from build123d import *

# Parameters (mm, degrees)
SKETCH_2_R          = 1.67
CUT_EXTRUDE_1_DEPTH = 10.939185077


with BuildPart() as part:
    # 草图1 → 旋转1 (revolve)
    with BuildSketch(Plane.XY, mode=Mode.PRIVATE) as revolve_1_sk:
        Polygon((0, 0), (3.12, 0), (3.12, 5.36), (3.93, 5.36), (3.93, 6.14), (3.12, 6.14), (3.12, 8.24), (0, 8.24), align=None)
    revolve(revolve_1_sk.sketch.rotate(Axis((0, 0, 0), (0, 1, 0)), 90), axis=Axis((0, 0, 0), (0, 1, 0)))

    # 草图2 → 切除-拉伸1 (cut, through all)
    with BuildSketch(Plane.XZ):
        with Locations(Location((0, 0, 0), (0, 0, 270))):
            Circle(SKETCH_2_R)
    extrude(amount=-CUT_EXTRUDE_1_DEPTH, mode=Mode.SUBTRACT)

    # 草图4 → 切除-旋转1 (revolve, cut)
    with BuildSketch(Plane.XY, mode=Mode.PRIVATE) as cut_revolve_1_sk:
        Polygon((2.62, 0), (1.67, 0.95), (0, 0.95), (0, 0), align=None)
        Polygon((2.62, 8.24), (1.67, 7.29), (0, 7.29), (0, 8.24), align=None)
    revolve(cut_revolve_1_sk.sketch.rotate(Axis((0, 0, 0), (0, -1, 0)), 90), axis=Axis((0, 0, 0), (0, -1, 0)), mode=Mode.SUBTRACT)


solid = part.part
Verification items for the finished model (mm, model axes). A direction names the side the tool comes from. Give positions to 0.01 mm unless a question says otherwise; leave off trailing zeros. Loops run counter-clockwise (first coordinate to the right, second up) from the corner with the lowest first, then second, coordinate; pieces in that order, holes last.
1. Cross-section at D-D on x = 2.75. Record the cut outline in (y, z).
Derived:
outline: (0, -1.47) - (5.36, -1.47) - (5.36, -2.81) - (6.14, -2.81) - (6.14, -1.47) - (8.24, -1.47) - (8.24, 1.47) - (6.14, 1.47) - (6.14, 2.81) - (5.36, 2.81) - (5.36, 1.47) - (0, 1.47) - close
2. Tool access check on faces 1 (the flat face through (-2, 8.24, 2)), 2 (the cylindrical face through (-0.937, 7.205, -2.976)), 3 (the cylindrical face through (-0.937, 2.718, -2.976)). Record the directions out of +Z, -Z, +X, -X, +Y, -Y that give a thin tool (end or side, any length) a straight path to the whole face; none if there is none.
Derived:
face 1: +Z, -Z, +X, -X, +Y
face 2: +Y
face 3: -Y
3. Release check for a two-part mould opening along Z. For faces 4 (the cylindrical face through (3.837, 5.755, 0.852)), 5 (the flat face through (-2, 0, -2)), 6 (the cylindrical face through (0.502, 4.076, -1.593)) record: +Z half, -Z half, draft (parallel to the pull), parting line (faces both ways), or undercut.
Derived:
face 4: parting line
face 5: draft
face 6: undercut
4. Cross-section at A-A on x = 0. Record the cut outline in (y, z), and give its area (3 significant figures).
Derived:
outline: (0, -3.12) - (5.36, -3.12) - (5.36, -3.93) - (6.14, -3.93) - (6.14, -3.12) - (8.24, -3.12) - (8.24, -2.62) - (7.29, -1.67) - (0.95, -1.67) - (0, -2.62) - close; (0, 2.62) - (0.95, 1.67) - (7.29, 1.67) - (8.24, 2.62) - (8.24, 3.12) - (6.14, 3.12) - (6.14, 3.93) - (5.36, 3.93) - (5.36, 3.12) - (0, 3.12) - close
area: 23.4 mm2
5. Go/stop test with flat-tipped pins: P1, Ø4, axis at x = 0, z = 0, coming from the -Y side; P2, Ø2, axis at x = -1, y = 2, coming from the -Z side; P3, Ø4, axis at x = 0, z = -0.5, coming from the -Y side. Record where each tip stops, or that it passes through.
Derived:
P1: stops at y = 0.62
P2: stops at z = -3.12
P3: stops at y = 0.12
6. Cross-section at B-B on z = 0. Record the cut outline in (x, y).
Derived:
outline: (-3.93, 5.36) - (-3.12, 5.36) - (-3.12, 0) - (-2.62, 0) - (-1.67, 0.95) - (-1.67, 7.29) - (-2.62, 8.24) - (-3.12, 8.24) - (-3.12, 6.14) - (-3.93, 6.14) - close; (1.67, 0.95) - (2.62, 0) - (3.12, 0) - (3.12, 5.36) - (3.93, 5.36) - (3.93, 6.14) - (3.12, 6.14) - (3.12, 8.24) - (2.62, 8.24) - (1.67, 7.29) - close
7. Cross-section at C-C on y = 4.5. Record the cut outline in (x, z).
Derived:
outline: circle Ø6.24 at (0, 0); hole circle Ø3.34 at (0, 0)
8. Material ranges on probe 1 along X at (y, z) = (3.25, 0); probe 2 along Z at (x, y) = (-0.5, 3.25); probe 3 along Y at (x, z) = (2.25, -2.5), recorded low to high.
Derived:
probe 1: x = -3.12 to -1.67, 1.67 to 3.12
probe 2: z = -3.08 to -1.59, 1.59 to 3.08
probe 3: y = 5.36 to 6.14
